Geometry check sheet. Reference: the model listing, model coordinates, mm. A direction names the side the tool comes from. Give positions to 0.01 mm unless a question says otherwise; leave off trailing zeros. Loops run counter-clockwise (first coordinate to the right, second up) from the corner with the lowest first, then second, coordinate; pieces in that order, holes last. Notation, with made-up numbers: (-2.5, 29) - (44.5, 29) arc R17 cw to (44.5, 33) - close; hole circle Ø10 at (-30.5, 25). An arc over 180 degrees is marked (long way). Write item = value, one per line. Start each with the question number.
from build123d import *

# Parameters (mm, degrees)
F1_DEPTH       = 38.1
F3_DEPTH       = 25.4
F4_W           = 71.12
F4_H           = 11.5075405073
F5_DEPTH       = 166.5568947792
F6_W           = 71.12
F6_H           = 51.0108690095
F7_DEPTH       = 24.13
F9_DEPTH       = 69.85
F11_DEPTH      = 25.4
F13_DEPTH      = 69.9950531125
F14_W          = 54.5549456358
F14_H          = 63.5
F15_DEPTH      = 9.9698379636
F17_DEPTH      = 79.6777680516
F19_DEPTH      = 169.2734211683
F20_W          = 25.5475714803
F20_H          = 57.1575462818
F21_DEPTH      = 79.7184870968
F21_DEPTH_BACK = 25.4
F22_W          = 28.8064163178
F22_H          = 50.0078629702
F23_DEPTH      = 6.35
F24_W          = 48.9942021668
F24_H          = 5.9489458799
F25_DEPTH      = 69.851
F26_W          = 20.0615301728
F26_H          = 66.6889064014
F27_DEPTH      = 25.4
F29_DEPTH      = 50.8
F31_DEPTH      = 86.3181352615
F32_W          = 21.5430464596
F32_H          = 13.2329052007
F33_DEPTH      = 43.8010953367
F34_R          = 4.2353424769
F34_R_2        = 4.016178265
F34_R_3        = 4.1045612078
F34_R_4        = 4.2518599003
F35_DEPTH      = 25.4


with BuildPart() as f1:
    # F0 (on Front) → F1 (new body, symmetric)
    with BuildSketch(Plane.XZ):
        Polygon((-22.1669822931, 56.0908690095), (-48.7866848707, 56.0908690095), (-48.7866848707, 0), (-29.5187681913, 0), (-29.5187681913, -55.6436777115), (-11.0080987215, -55.6436777115), (-11.0080987215, -14.1748189926), (22.619381547, 15.2303725481), (67.2549456358, 15.2303725481), (67.2549456358, 31.8179130554), (0, 31.8179130554), (-22.1669822931, 44.9371486902), align=None)
    extrude(amount=F1_DEPTH, both=True)

    # F2 (on face) → F3 (cut)
    with BuildSketch(Plane.XZ.offset(38.1)):
        Polygon((64.7149456358, 17.7703725481), (64.7149456358, 29.2779130554), (-0.6953087103, 29.2779130554), (-24.7069822931, 43.4889048609), (-24.7069822931, 53.5508690095), (-46.2466848707, 53.5508690095), (-46.2466848707, 2.54), (-26.9787681913, 2.54), (-26.9787681913, -53.1036777115), (-13.5480987215, -53.1036777115), (-13.5480987215, -13.0217612085), (21.665474667, 17.7703725481), align=None)
    extrude(amount=-F3_DEPTH, mode=Mode.SUBTRACT)

    # F4 (on face) → F5 (cut)
    with BuildSketch(Plane.YZ.offset(67.2549456358)):
        with Locations((0, 23.5241428018)):
            Rectangle(F4_W, F4_H)
    extrude(amount=-F5_DEPTH, mode=Mode.SUBTRACT)

    # F6 (on face) → F7 (cut)
    with BuildSketch(Plane(origin=(-48.7866848707, 0, 0), x_dir=(0, -1, 0), z_dir=(-1, 0, 0))):
        with Locations((0, 28.0454345047)):
            Rectangle(F6_W, F6_H)
    extrude(amount=-F7_DEPTH, mode=Mode.SUBTRACT)

    # F8 (on face) → F9 (cut)
    with BuildSketch(Plane.XY.offset(17.7703725481)):
        Polygon((-22.1166848707, -33.02), (24.205474667, -33.02), (24.205474667, -35.56), (64.7149456358, -35.56), (64.7149456358, 33.02), (-22.1166848707, 33.02), align=None)
    extrude(amount=-F9_DEPTH, mode=Mode.SUBTRACT)

    # F10 (on face) → F11 (cut)
    with BuildSketch(Plane(origin=(0, 38.1, 0), x_dir=(-1, 0, 0), z_dir=(0, 1, 0))):
        Polygon((-64.7149456358, 17.7703725481), (-21.665474667, 17.7703725481), (13.5480987215, -13.0217612085), (13.5480987215, -53.1036777115), (26.9787681913, -53.1036777115), (26.9787681913, 2.54), (46.2466848707, 2.54), (46.2466848707, 53.5508690095), (24.7069822931, 53.5508690095), (24.7069822931, 43.4889048609), (0.6953087103, 29.2779130554), (-64.7149456358, 29.2779130554), align=None)
    extrude(amount=-F11_DEPTH, mode=Mode.SUBTRACT)

    # F12 (on face) → F13 (join)
    with BuildSketch(Plane(origin=(0, -33.02, 0), x_dir=(-1, 0, 0), z_dir=(0, 1, 0))):
        Polygon((-21.665474667, 17.7703725481), (-24.205474667, 17.7703725481), (-24.205474667, 15.2303725481), (-22.619381547, 15.2303725481), (-22.6041972144, 15.2170947704), (-22.5458946079, 15.2166113257), (-20.4890360799, 13.3675146709), (-20.4890360799, 16.7416483703), align=None)
    extrude(amount=F13_DEPTH)

    # F14 (on face) → F15 (join)
    with BuildSketch(Plane.XY.offset(31.8179130554)):
        with Locations((33.6274728179, 0)):
            Rectangle(F14_W, F14_H)
    extrude(amount=F15_DEPTH)

    # F16 (on face) → F17 (join)
    with BuildSketch(Plane.XY.offset(41.787751019)):
        Polygon((12.1729150414, -26.1881239712), (54.4057376683, -26.1881239712), (54.4057376683, 11.6354003549), (44.7186082602, 11.6354003549), (44.7186082602, -10.164026171), (30.9308022261, -10.164026171), (30.9308022261, 24.1416729987), (22.2798474133, 24.1416729987), (22.2798474133, 0), (12.1729150414, 0), align=None)
    extrude(amount=F17_DEPTH)

    # F18 (on face) → F19 (cut)
    with BuildSketch(Plane.XZ.offset(26.1881239712)):
        Polygon((27.9768835753, 109.9416464567), (19.3683411926, 109.9416464567), (19.3683411926, 47.6811267436), (48.9032641053, 47.6811267436), (48.9032641053, 109.9416464567), (40.2469709516, 109.9416464567), (40.2469709516, 58.1681281328), (27.9768835753, 58.1681281328), align=None)
    extrude(amount=-F19_DEPTH, mode=Mode.SUBTRACT)

    # F20 (on face) → F21 (cut, two sides)
    with BuildSketch(Plane.YZ.offset(30.9308022261)) as f21_sk:
        with Locations((6.7332647741, 90.1354327798)):
            Rectangle(F20_W, F20_H)
    extrude(amount=-F21_DEPTH, mode=Mode.SUBTRACT)
    extrude(f21_sk.sketch, amount=F21_DEPTH_BACK, mode=Mode.SUBTRACT)

    # F22 (on face) → F23 (cut)
    with BuildSketch(Plane(origin=(0, 0, 29.2779130554), x_dir=(1, 0, 0), z_dir=(0, 0, -1))):
        with Locations((45.0015263632, 4.0960470214)):
            Rectangle(F22_W, F22_H)
    extrude(amount=-F23_DEPTH, mode=Mode.SUBTRACT)

    # F24 (on face) → F25 (cut, through all)
    with BuildSketch(Plane(origin=(0, 31.75, 0), x_dir=(-1, 0, 0), z_dir=(0, 1, 0))):
        with Locations((-33.5451457649, 36.8936993182)):
            Rectangle(F24_W, F24_H)
    extrude(amount=-F25_DEPTH, mode=Mode.SUBTRACT)

    # F26 (on face) → F27 (cut)
    with BuildSketch(Plane.XY.offset(56.0908690095)):
        with Locations((-35.4243777692, -0.5888808519)):
            Rectangle(F26_W, F26_H)
    extrude(amount=-F27_DEPTH, mode=Mode.SUBTRACT)

    # F28 (on face) → F29 (join)
    with BuildSketch(Plane.YZ.offset(-26.9787681913)):
        with BuildLine():
            Line((29.8926215619, -48.8248394649), (29.8926215619, -26.276535997))
            ThreePointArc((29.8926215619, -26.276535997), (20.0002810954, -18.0048741229), (18.7791224223, -30.8418348831))
            Line((18.7791224223, -30.8418348831), (18.7791224223, -48.8248394649))
            Line((18.7791224223, -48.8248394649), (29.8926215619, -48.8248394649))
        make_face()
    extrude(amount=F29_DEPTH)

    # F30 (on face) → F31 (cut)
    with BuildSketch(Plane.YZ.offset(23.8212318087)):
        with BuildLine():
            Line((21.3191224223, -46.2848394649), (27.3526215619, -46.2848394649))
            Line((27.3526215619, -46.2848394649), (27.3526215619, -25.9773227743))
            ThreePointArc((27.3526215619, -25.9773227743), (20.4981967379, -20.5767900682), (21.3191224223, -29.2644234743))
            Line((21.3191224223, -29.2644234743), (21.3191224223, -46.2848394649))
        make_face()
    extrude(amount=-F31_DEPTH, mode=Mode.SUBTRACT)

    # F32 (on face) → F33 (join)
    with BuildSketch(Plane(origin=(-24.6566848707, 0, 0), x_dir=(0, -1, 0), z_dir=(-1, 0, 0))):
        with Locations((-0.0923750922, 9.1564526004)):
            Rectangle(F32_W, F32_H)
    extrude(amount=F33_DEPTH)

    # F34 (on face) → F35 (cut)
    with BuildSketch(Plane(origin=(0, 10.863898322, 0), x_dir=(-1, 0, 0), z_dir=(0, 1, 0))):
        with Locations((30.2229300141, 8.5582211614)):
            Circle(F34_R)
        with Locations((40.7767370343, 8.5658058524)):
            Circle(F34_R_2)
        with Locations((51.4430738986, 8.8405385613)):
            Circle(F34_R_3)
        with Locations((62.559530139, 9.0516358614)):
            Circle(F34_R_4)
    extrude(amount=-F35_DEPTH, mode=Mode.SUBTRACT)


solid = f1.part
1) Cross-section at A-A on z = 22. Enter the section's corners in (x, y), and give its area (3 significant figures).
2) Material ranges on line 1 along X through (y, z) = (-8.5, 75.5); line 2 along Z through (x, y) = (33.5, 29.5); line 3 along Z through (x, y) = (-51, -10), recorded low to high.
3) Release check for a two-part mould opening along X. For faces 1 (the face through (-48.787, 0, 55)), 2 (the face through (-7, -33.02, -10)), 3 (the face through (58.042, 0, 38)), 4 (the face through (54.406, -12, 72)) record: pulls with the +X half, pulls with the -X half, needs draft (parallel to the pull), parting line crosses it, or undercut.
4) Tool access check on faces 5 (the face through (6.35, 0, 37)), 6 (the face through (30.931, 20, 85)), 7 (the face through (45, -29.1, 32)), 8 (the face through (-20, -26, -53.104)), 9 (the face through (9.048, 0, 37)). Record the directions out of +Z, -Z, +X, -X, +Y, -Y that give a thin tool (end or side, any length) a straight path to the whole face; none if there is none.
5) Cross-section at C-C on z = -35. Enter the section's corners in (x, y), and give its area (3 significant figures).
6) Cross-section at B-B on y = -17. Give the number of separate pieces and of enclosed holes in the cut face, and give its area (3 significant figures).
7) Gauge pin test, flat ends, axial feed: P1, Ø7.5, axis at y = 23.5, z = -35.5, coming from the +X side; P2, Ø7, axis at x = 27, z = 94, coming from the -Y side; P3, Ø12.5, axis at y = 12, z = 115, coming from the -X side; P4, Ø8, axis at x = 10.5, z = 18.5, coming from the +Y side. Record the tip position at first contact, or that the pin passes through.
Checked values:
q1.outline = (-48.79, -38.1) - (-46.25, -38.1) - (-46.25, -35.56) - (-48.79, -35.56) - close; (-48.79, 35.56) - (-46.25, 35.56) - (-46.25, 38.1) - (-48.79, 38.1) - close; (64.71, -38.1) - (67.25, -38.1) - (67.25, -35.56) - (64.71, -35.56) - close; (64.71, 35.56) - (67.25, 35.56) - (67.25, 38.1) - (64.71, 38.1) - close
q1.area = 25.8 mm²
q2.line_1 = 12.17 to 19.37, 27.98 to 30.93, 48.9 to 54.41
q2.line_2 = 29.28 to 33.92, 39.87 to 41.79
q2.line_3 = 2.54 to 4.76, 12.92 to 15.77
q3.face_1 = pulls with the -X half
q3.face_2 = needs draft
q3.face_3 = undercut
q3.face_4 = pulls with the +X half
q4.face_5 = +Z, +Y, -Y
q4.face_6 = +Z, +Y
q4.face_7 = -Z
q4.face_8 = -Y
q4.face_9 = +Y, -Y
q5.outline = (-29.52, -38.1) - (-26.98, -38.1) - (-26.98, -12.7) - (-22.12, -12.7) - (-22.12, 12.7) - (-26.98, 12.7) - (-26.98, 18.78) - (23.82, 18.78) - (23.82, 21.32) - (-29.52, 21.32) - close; (-29.52, 27.35) - (23.82, 27.35) - (23.82, 29.89) - (-26.98, 29.89) - (-26.98, 38.1) - (-29.52, 38.1) - close; (-13.55, -38.1) - (-11.01, -38.1) - (-11.01, -33.02) - (-13.55, -33.02) - close; (-13.55, 33.02) - (-11.01, 33.02) - (-11.01, 38.1) - (-13.55, 38.1) - close
q5.area = 586 mm²
q6.separate_pieces = 5
q6.enclosed_holes = 1
q6.area = 2,810 mm²
q7.P1 = 23.82
q7.P2 = -26.19
q7.P3 = 22.28
q7.P4 = through
